from build123d import *

# Parameters (mm, degrees)
SKETCH1_W           = 40
SKETCH1_H           = 20
BOSS_EXTRUDE1_DEPTH = 38
SKETCH2_W           = 20
SKETCH2_H           = 4
BOSS_EXTRUDE2_DEPTH = 27
SKETCH3_R           = 2.5
CUT_EXTRUDE5_DEPTH  = 53.6
SKETCH4_R           = 7.5
BOSS_EXTRUDE3_DEPTH = 2
BOSS_EXTRUDE3_TAPER = 39
SKETCH5_R           = 3.5
BOSS_EXTRUDE4_DEPTH = 5.2
SKETCH6_R           = 10
BOSS_EXTRUDE5_DEPTH = 2
FILLET1_R           = 2
SKETCH7_R           = 2.5
SKETCH7_R_2         = 1
CUT_EXTRUDE9_DEPTH  = 6


with BuildPart() as part:
    # Sketch1 → Boss-Extrude1 (new body)
    with BuildSketch(Plane(origin=(0, 0, 0), x_dir=(1, 0, 0), z_dir=(0, 1, 0))):
        Rectangle(SKETCH1_W, SKETCH1_H)
    extrude(amount=BOSS_EXTRUDE1_DEPTH)

    # Sketch2 → Boss-Extrude2 (add, symmetric)
    with BuildSketch(Plane(origin=(0, 0, 0), x_dir=(0, 0, -1), z_dir=(1, 0, 0))):
        with Locations((0, 30)):
            Rectangle(SKETCH2_W, SKETCH2_H)
    extrude(amount=BOSS_EXTRUDE2_DEPTH, both=True)

    # Sketch3 → Cut-Extrude5 (cut)
    with BuildSketch(Plane(origin=(0, 32, 0), x_dir=(1, 0, 0), z_dir=(0, 1, 0))):
        with Locations(Location((24.4, 5, 0), (0, 0, 270))):
            Circle(SKETCH3_R)
        with Locations(Location((24.4, -5, 0), (0, 0, 270))):
            Circle(SKETCH3_R)
    cut_extrude5 = extrude(amount=-CUT_EXTRUDE5_DEPTH, mode=Mode.SUBTRACT)

    # Mirror1: Cut-Extrude5 across plane
    add(cut_extrude5.mirror(Plane(origin=(0, 0, 0), x_dir=(0, 0, 1), z_dir=(1, 0, 0))), mode=Mode.SUBTRACT)

    # Sketch4 → Boss-Extrude3 (add)
    with BuildSketch(Plane(origin=(0, 38, 0), x_dir=(1, 0, 0), z_dir=(0, 1, 0))):
        with Locations((10, 0)):
            Circle(SKETCH4_R)
    extrude(amount=BOSS_EXTRUDE3_DEPTH, taper=BOSS_EXTRUDE3_TAPER)

    # Sketch5 → Boss-Extrude4 (add)
    with BuildSketch(Plane(origin=(0, 40, 0), x_dir=(1, 0, 0), z_dir=(0, 1, 0))):
        with Locations(Location((10, 0, 0), (0, 0, 270))):
            Circle(SKETCH5_R)
    extrude(amount=BOSS_EXTRUDE4_DEPTH)

    # Sketch6 → Boss-Extrude5 (add)
    with BuildSketch(Plane(origin=(0, 45.2, 0), x_dir=(1, 0, 0), z_dir=(0, 1, 0))):
        with Locations(Location((10, 0, 0), (0, 0, 270))):
            Circle(SKETCH6_R)
    extrude(amount=BOSS_EXTRUDE5_DEPTH)

    # Fillet1
    fillet1_edges = [part.edges().sort_by_distance(p)[0] for p in [
        (-27, 30, -10),
        (-27, 30, 10),
        (27, 30, -10),
        (27, 30, 10),
    ]]
    fillet(fillet1_edges, radius=FILLET1_R)

    # Sketch7 → Cut-Extrude9 (cut)
    with BuildSketch(Plane(origin=(0, 47.2, 0), x_dir=(1, 0, 0), z_dir=(0, 1, 0))):
        with Locations(Location((10, 0, 0), (0, 0, 270))):
            Circle(SKETCH7_R)
        with Locations(Location((10, 7, 0), (0, 0, 270))):
            Circle(SKETCH7_R_2)
        with Locations(Location((13, 7, 0), (0, 0, 270))):
            Circle(SKETCH7_R_2)
        with Locations(Location((7, 7, 0), (0, 0, 270))):
            Circle(SKETCH7_R_2)
        with Locations(Location((17, 3, 0), (0, 0, 270))):
            Circle(SKETCH7_R_2)
        with Locations(Location((17, 0, 0), (0, 0, 270))):
            Circle(SKETCH7_R_2)
        with Locations(Location((17, -3, 0), (0, 0, 270))):
            Circle(SKETCH7_R_2)
        with Locations(Location((13, -7, 0), (0, 0, 270))):
            Circle(SKETCH7_R_2)
        with Locations(Location((10, -7, 0), (0, 0, 270))):
            Circle(SKETCH7_R_2)
        with Locations(Location((7, -7, 0), (0, 0, 270))):
            Circle(SKETCH7_R_2)
        with Locations(Location((3, -3, 0), (0, 0, 270))):
            Circle(SKETCH7_R_2)
        with Locations(Location((3, 0, 0), (0, 0, 270))):
            Circle(SKETCH7_R_2)
        with Locations(Location((3, 3, 0), (0, 0, 270))):
            Circle(SKETCH7_R_2)
    extrude(amount=-CUT_EXTRUDE9_DEPTH, mode=Mode.SUBTRACT)


solid = part.part
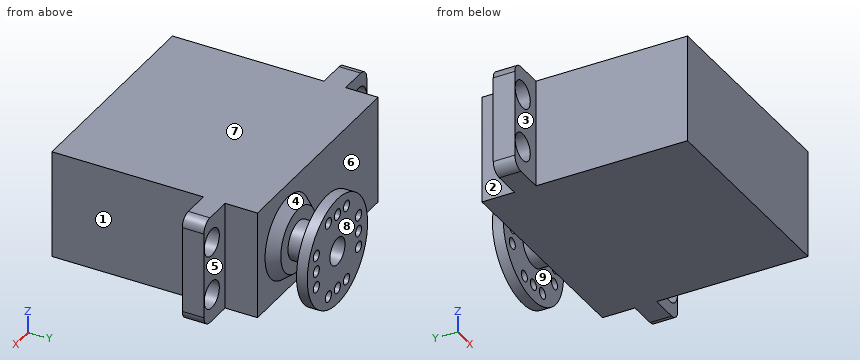
Check sheet for the modelled part. Datum: model origin and axes. Units: mm. Face numbers are marked on the shaded views. A direction names the side the tool comes from. Give positions to 0.01 mm unless a question says otherwise; leave off trailing zeros. Write each loop counter-clockwise with the first axis right and the second up, starting at its lowest first coordinate (ties: lowest second). Pieces come first, ordered by that corner, then holes. Notation, with made-up numbers: (39.25, 8) -> (72.25, 8) arc R18 ccw to (72.25, 19) -> close; hole circle Ø6 at (-18, 26.25). An arc over 180 degrees is marked (long way). One line per item, written item: value. Start each with the question number.
Item 1: Section check B-B on y = 43. Record the cut outline in (x, z), then the cut area to 3 significant figures.
Item 2: Section check C-C on x = -2.5. Record the cut outline in (y, z), then the cut area to 3 significant figures.
Item 3: Draft check along Y on the marked faces 6, 7, 8 and 9. Enter one of: +Y half, -Y half, draft (parallel to the pull), parting line (faces both ways), or undercut.
Item 4: Section check A-A on x = -24.4. Record the cut outline in (y, z), then the cut area to 3 significant figures.
Item 5: Material ranges on probe 1 along Y at (x, z) = (8.5, 3.25); probe 2 along Y at (x, z) = (4, -7.5); probe 3 along X at (y, z) = (46.45, 3), recorded low to high. Write a range as from..to.
Item 6: Tool access check on the marked faces 1, 2, 3, 4 and 5. Record the directions out of +Z, -Z, +X, -X, +Y, -Y that give a thin tool (end or side, any length) a straight path to the whole face; none if there is none.
Item 7: Section check D-D on z = 5. State how many separate pieces and enclosed holes the cut face has, then the cut area to 3 significant figures.
Item 8: Gauge pin test, flat ends, axial feed: pin 1 (1.5 mm diameter, centred on x = 14, z = 7.5, fed in from -Y); pin 2 (10 mm diameter, centred on y = 10.5, z = 0.5, fed in from +X); pin 3 (1.6 mm diameter, centred on x = 17, z = 3, fed in from +Y); pin 4 (5 mm diameter, centred on x = -14.5, z = 4, fed in from +Y). Record the tip position at first contact, or that the pin passes through.
Results list:
1. outline: circle Ø7 at (10, 0); hole circle Ø5 at (10, 0)
1. area: 18.8 mm²
2. outline: (0, -10) -> (38, -10) -> (38, 10) -> (0, 10) -> close
2. area: 760 mm²
3. face 6: undercut
3. face 7: draft
3. face 8: +Y half
3. face 9: undercut
4. outline: (28, -10) -> (32, -10) -> (32, -7.5) -> (28, -7.5) -> close; (28, -2.5) -> (32, -2.5) -> (32, 2.5) -> (28, 2.5) -> close; (28, 7.5) -> (32, 7.5) -> (32, 10) -> (28, 10) -> close
4. area: 40.0 mm²
5. probe 1: 0..40, 45.2..47.2
5. probe 2: 0..38, 45.2..47.2
5. probe 3: 0.46..2, 4..16, 18..19.54
6. face 1: +Z, -Z, +X, -Y
6. face 2: +Z, -Z, -X, +Y
6. face 3: +Z, -Z, -X, -Y
6. face 4: none
6. face 5: +Z, -Z, +X, +Y
7. separate pieces: 4
7. enclosed holes: 0
7. area: 1,590 mm²
8. pin 1: y = 0
8. pin 2: x = 20
8. pin 3: y = 38.84
8. pin 4: y = 38
